```python
from build123d import *

# Parameters (mm, degrees)
F2_DEPTH  = 19.05
F3_W      = 85.725
F3_H      = 19.05
F3_R      = 117.475
F4_DEPTH  = 25.4
F5_W      = 152.4
F5_H      = 19.05
F6_DEPTH  = 25.4
F8_DEPTH  = 25.4
F9_W      = 19.05
F9_H      = 101.6
F10_DEPTH = 25.4
F12_DEPTH = 25.4


# Not quite as in the source:
# - a variable given as a bare number and used for a length is read in inches; the dataset says mm whatever the document's units were


with BuildPart() as f2:
    # F1 (on Front) → F2 (new body)
    with BuildSketch(Plane.XZ):
        with BuildLine():
            Line((355.6, 355.6), (203.2, 355.6))
            Line((203.2, 355.6), (-203.2, 355.6))
            Line((-203.2, 355.6), (-355.6, 355.6))
            ThreePointArc((-355.6, 355.6), (-331.3431214209, 216.6595631931), (-261.4423933195, 94.1576066805))
            ThreePointArc((-261.4423933195, 94.1576066805), (-222.3790342141, 0), (-261.4423933195, -94.1576066805))
            ThreePointArc((-261.4423933195, -94.1576066805), (-331.3431214209, -216.6595631931), (-355.6, -355.6))
            Line((-355.6, -355.6), (-203.2, -355.6))
            Line((-203.2, -355.6), (203.2, -355.6))
            Line((203.2, -355.6), (355.6, -355.6))
            ThreePointArc((355.6, -355.6), (331.3431214209, -216.6595631931), (261.4423933195, -94.1576066805))
            ThreePointArc((261.4423933195, -94.1576066805), (232.4074653208, 0), (261.4423933195, 94.1576066805))
            ThreePointArc((261.4423933195, 94.1576066805), (331.3431214209, 216.6595631931), (355.6, 355.6))
        make_face()
    extrude(amount=F2_DEPTH)

    # F3 (on face) → F4 (cut)
    with BuildSketch(Plane.XZ.offset(19.05)):
        with Locations((-312.7375, 346.075)):
            Rectangle(F3_W, F3_H)
        with Locations((312.7375, 346.075)):
            Rectangle(F3_W, F3_H)
        with Locations((312.7375, -346.075)):
            Rectangle(F3_W, F3_H)
        with Locations((-312.7375, -346.075)):
            Rectangle(F3_W, F3_H)
        with Locations((0, 355.6)):
            Circle(F3_R)
        with Locations((0, -355.6)):
            Circle(F3_R)
    extrude(amount=-F4_DEPTH, mode=Mode.SUBTRACT)

    # F5 (on face) → F6 (cut)
    with BuildSketch(Plane.XZ.offset(19.05)):
        with Locations((-193.675, 193.675)):
            Rectangle(F5_W, F5_H)
        with Locations((193.675, 193.675)):
            Rectangle(F5_W, F5_H)
    extrude(amount=-F6_DEPTH, mode=Mode.SUBTRACT)

    # F7 (on face) → F8 (cut)
    with BuildSketch(Plane.XZ.offset(19.05)):
        with BuildLine():
            Line((-250.825, 184.15), (-250.825, 203.2))
            ThreePointArc((-250.825, 203.2), (-260.35, 212.725), (-269.875, 203.2))
            Line((-269.875, 203.2), (-269.875, 184.15))
            ThreePointArc((-269.875, 184.15), (-260.35, 174.625), (-250.825, 184.15))
        make_face()
        with BuildLine():
            ThreePointArc((-117.475, 203.2), (-127, 212.725), (-136.525, 203.2))
            Line((-136.525, 203.2), (-136.525, 184.15))
            ThreePointArc((-136.525, 184.15), (-127, 174.625), (-117.475, 184.15))
            Line((-117.475, 184.15), (-117.475, 203.2))
        make_face()
        with BuildLine():
            Line((117.475, 203.2), (117.475, 184.15))
            ThreePointArc((117.475, 184.15), (127, 174.625), (136.525, 184.15))
            Line((136.525, 184.15), (136.525, 203.2))
            ThreePointArc((136.525, 203.2), (127, 212.725), (117.475, 203.2))
        make_face()
        with BuildLine():
            ThreePointArc((269.875, 203.2), (260.35, 212.725), (250.825, 203.2))
            Line((250.825, 203.2), (250.825, 184.15))
            ThreePointArc((250.825, 184.15), (260.35, 174.625), (269.875, 184.15))
            Line((269.875, 184.15), (269.875, 203.2))
        make_face()
    extrude(amount=-F8_DEPTH, mode=Mode.SUBTRACT)

    # F9 (on face) → F10 (cut)
    with BuildSketch(Plane.XZ.offset(19.05)):
        with Locations((260.35, 193.675)):
            Rectangle(F9_W, F9_H)
        with Locations((260.35, -193.675)):
            Rectangle(F9_W, F9_H)
    extrude(amount=-F10_DEPTH, mode=Mode.SUBTRACT)

    # F11 (on face) → F12 (cut)
    with BuildSketch(Plane.XZ.offset(19.05)):
        with BuildLine():
            Line((269.875, 244.475), (250.825, 244.475))
            ThreePointArc((250.825, 244.475), (241.3, 234.95), (250.825, 225.425))
            Line((250.825, 225.425), (269.875, 225.425))
            ThreePointArc((269.875, 225.425), (279.4, 234.95), (269.875, 244.475))
        make_face()
        with BuildLine():
            ThreePointArc((269.875, 142.875), (279.4, 152.4), (269.875, 161.925))
            Line((269.875, 161.925), (250.825, 161.925))
            ThreePointArc((250.825, 161.925), (241.3, 152.4), (250.825, 142.875))
            Line((250.825, 142.875), (269.875, 142.875))
        make_face()
        with BuildLine():
            Line((269.875, -142.875), (250.825, -142.875))
            ThreePointArc((250.825, -142.875), (241.3, -152.4), (250.825, -161.925))
            Line((250.825, -161.925), (269.875, -161.925))
            ThreePointArc((269.875, -161.925), (279.4, -152.4), (269.875, -142.875))
        make_face()
        with BuildLine():
            ThreePointArc((250.825, -225.425), (241.3, -234.95), (250.825, -244.475))
            Line((250.825, -244.475), (269.875, -244.475))
            ThreePointArc((269.875, -244.475), (279.4, -234.95), (269.875, -225.425))
            Line((269.875, -225.425), (250.825, -225.425))
        make_face()
    extrude(amount=-F12_DEPTH, mode=Mode.SUBTRACT)


solid = f2.part
```
Design review of the part built by this model. Coordinates are the model's own, in mm. A direction names the side the tool comes from. Give positions to 0.01 mm unless a question says otherwise; leave off trailing zeros. Loops run counter-clockwise (first coordinate to the right, second up) from the corner with the lowest first, then second, coordinate; pieces in that order, holes last. Notation, with made-up numbers: (50.5, 55) -> (98.5, 55) arc R19 cw to (98.5, 88) -> close; hole circle Ø10 at (-18, 77). An arc over 180 degrees is marked (long way). One line per item, written item: value.
Q1. We need section A-A on x = 198. Give the boundary of the cut face in (y, z).
Numbers:
outline: (-19.05, -355.6) -> (0, -355.6) -> (0, 184.15) -> (-19.05, 184.15) -> close; (-19.05, 203.2) -> (0, 203.2) -> (0, 355.6) -> (-19.05, 355.6) -> close
Q2. We need section C-C on x = 0. Give the boundary of the cut face in (y, z) (3 decimals).
Numbers:
outline: (-19.05, -238.125) -> (0, -238.125) -> (0, 238.125) -> (-19.05, 238.125) -> close
Q3. We need section D-D on y = -6.5. Give the number of separate pieces and of enclosed holes in the cut face, and give its area (3 significant figures).
Numbers:
separate pieces: 1
enclosed holes: 3
area: 369,000 mm^2
Q4. Machinability: for faces 1 (the flat face through (-269.875, -10, -346)), 2 (the cylindrical face through (126.791, -9.658, 174.627)), 3 (the flat face through (-313, -10, 336.55)), which of the approach directions +Z, -Z, +X, -X, +Y, -Y give a long, thin tool a straight path to every point of the face, cutting with its end or side? Answer none if there is none.
Numbers:
face 1: -Z, -X, +Y, -Y
face 2: +Y, -Y
face 3: +Z, -X, +Y, -Y
Q5. For L1, parallel to Z at x = 161.5, y = -9.25; L2, parallel to Z at x = 251.5, y = -14.5 (3 decimals); L3, parallel to Z at x = 257.5, y = -14.75 (3 decimals), list the stretches that pass through material, from the lowest coordinate up.
Numbers:
L1: z = -355.6 to 184.15, 203.2 to 355.6
L2: z = -355.6 to -244.475, -142.875 to -77.586, 77.586 to 142.875, 244.475 to 355.6
L3: z = -355.6 to -244.475, -142.875 to -88.095, 88.095 to 142.875, 244.475 to 355.6
Q6. For pin 1 Ø9.5 at (y, z) = (-11, 178) entering from +X; pin 2 Ø5.5 at (x, y) = (299, -13) entering from +Z; pin 3 Ø9.5 at (y, z) = (-12, 208) entering from -X, all flat-tipped, find the tip position at first contact; note any pin that passes through.
Numbers:
pin 1: stops at x = 317.39
pin 2: stops at z = 336.55
pin 3: stops at x = -329.91
Q7. We need section B-B on z = -152.4. Give the boundary of the cut face in (x, y), and give its area (3 significant figures).
Numbers:
outline: (-301.71, -19.05) -> (241.3, -19.05) -> (241.3, 0) -> (-301.71, 0) -> close; (279.4, -19.05) -> (301.71, -19.05) -> (301.71, 0) -> (279.4, 0) -> close
area: 10,800 mm^2
